Drawing for the job (mm, zero at the part's lowest x, y, z). Coordinates: 2 decimals unless noted, no trailing zeros. Loops run counter-clockwise (first coordinate to the right, second up) from the corner with the lowest first, then second, coordinate; pieces in that order, holes last. Notation, with made-up numbers: (66, 89.25) -> (85, 89.25) arc R13 ccw to (85, 93.25) -> close; hole circle Ø2 at (41.5, -4). An arc over 180 degrees is marked (long way). Write item = value, one per line. Start each with the question number.
(1) Band-saw the part on B-B (y = 1.25). Write the cut outline in (x, z).
(2) Band-saw the part on C-C (y = 8.5). Write the cut outline in (x, z) (1 decimal).
(3) Band-saw the part on A-A (y = 7.5). Write the cut outline in (x, z), and give its area (3 significant figures).
(4) Drill centre lines: line 1 (X direction, y = 7, z = 6.5) (1 decimal); line 2 (X direction, y = 8.25, z = 7.25) (1 decimal); line 3 (Y direction, x = 4.25, z = 4.25). Where is each one in solid material? Low to high. Write a range as from..to.
(5) Flat gauge pins, fed straight in: P1, Ø1, axis at y = 2, z = 5, coming from the -X side (1 decimal); P2, Ø1, axis at x = 4.5, z = 2, coming from the +Y side. Where does each tip first touch, or does it go through?
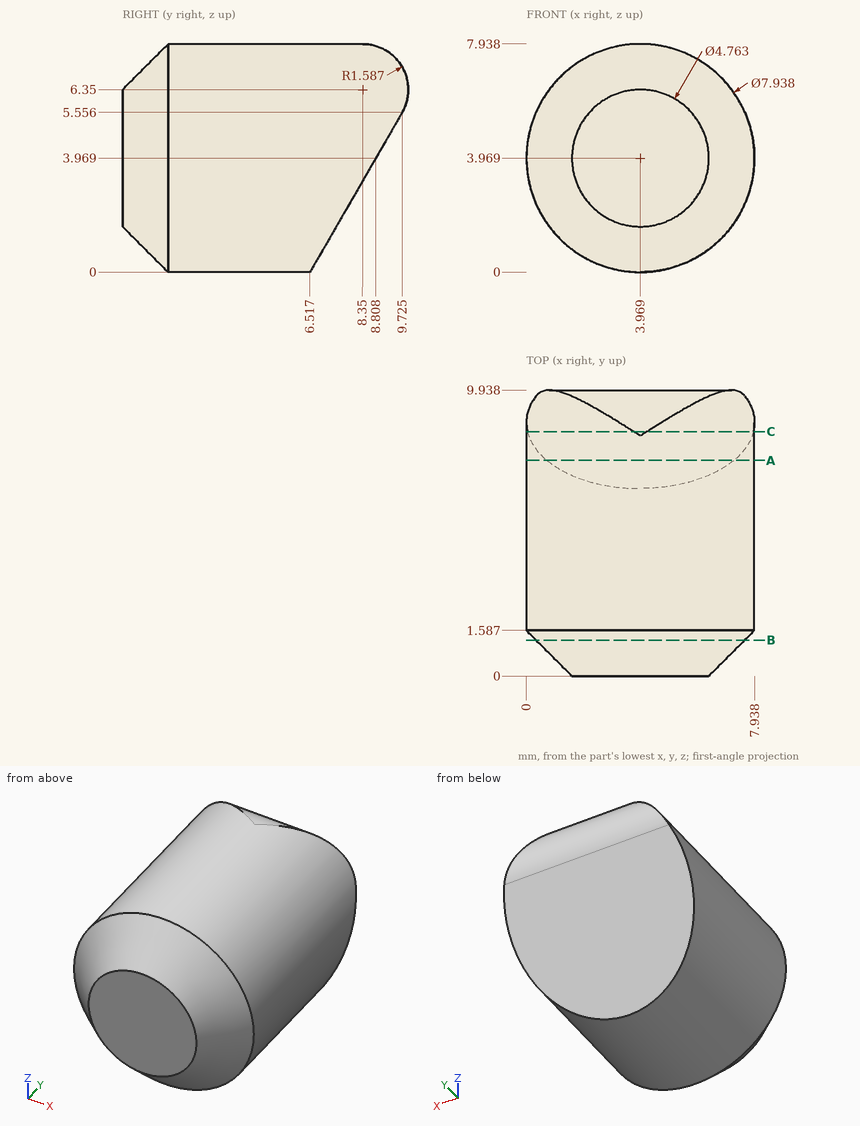
Findings below:
q1.outline = circle Ø7.26 at (3.97, 3.97)
q2.outline = (0, 3.4) -> (7.9, 3.4) arc R4 ccw to (4.2, 7.9) -> (3.7, 7.9) arc R4 ccw to start
q3.outline = (0.71, 1.7) -> (7.23, 1.7) arc R3.97 ccw (long way) to start
q3.area = 41.7 mm²
q4.line_1 = 0.9..7
q4.line_2 = 1.7..6.2
q4.line_3 = 0..8.97
q5.P1 = 0
q5.P2 = 7.96
